```python
from build123d import *

# Parameters (mm, degrees)
PAD_DEPTH    = 15
SKETCH001_R  = 2
POCKET_DEPTH = 5
CHAMFER_SIZE = 1
FILLET_R     = 1


with BuildPart() as part:
    # Sketch → Pad (new body)
    with BuildSketch(Plane.XY):
        with BuildLine():
            Line((13, -10), (-35, -10))
            ThreePointArc((-35, 15), (-47.5, 2.5), (-35, -10))
            Line((-35, 15), (0, 15))
            Line((0, 15), (0, 0))
            Line((0, 0), (-5, 0))
            Line((-5, 0), (-5, 10))
            Line((-5, 10), (-35, 10))
            ThreePointArc((-35, 10), (-42.499997, 2.5), (-35, -5))
            Line((-35, -5), (13, -5))
            Line((13, -5), (13, -10))
        make_face()
    extrude(amount=PAD_DEPTH)

    # Sketch001 (on Face9 of Pad) → Pocket (cut)
    with BuildSketch(Plane(origin=(0, -5, 0), x_dir=(-1, 0, 0), z_dir=(0, 1, 0))):
        with Locations((-8, 7.5)):
            Circle(SKETCH001_R)
    extrude(amount=-POCKET_DEPTH, mode=Mode.SUBTRACT)

    # Chamfer
    chamfer_edges = [part.edges().sort_by_distance(p)[0] for p in [
        (10, -5, 7.5),
    ]]
    chamfer(chamfer_edges, length=CHAMFER_SIZE)

    # Fillet
    fillet_edges = [part.edges().sort_by_distance(p)[0] for p in [
        (-11, -10, 0),
        (13, -7.5, 0),
        (-11, -5, 0),
        (-20, 10, 0),
        (-5, 5, 0),
        (-2.5, 0, 0),
        (0, 7.5, 0),
        (13, -5, 7.5),
        (-11, -5, 15),
        (-17.5, 15, 0),
        (0, 15, 7.5),
        (-17.5, 15, 15),
        (-47.5, 2.5, 0),
        (-42.499997, 2.5, 0),
        (-47.5, 2.5, 15),
        (-20, 10, 15),
        (-42.499997, 2.5, 15),
        (-5, 5, 15),
        (-2.5, 0, 15),
        (0, 7.5, 15),
        (13, -7.5, 15),
        (-11, -10, 15),
        (-5, 0, 7.5),
        (0, 0, 7.5),
        (13, -10, 7.5),
    ]]
    fillet(fillet_edges, radius=FILLET_R)


solid = part.part
```
Part model, mm, in its own coordinate system. A direction names the side the tool comes from. Coordinates: 2 decimals unless noted, no trailing zeros. Loops run counter-clockwise (first coordinate to the right, second up) from the corner with the lowest first, then second, coordinate; pieces in that order, holes last. Notation, with made-up numbers: (-31.75, -9.5) - (16.25, -9.5) arc R12 cw to (16.25, 11.5) - close; hole circle Ø6 at (34.25, 34). An arc over 180 degrees is marked (long way). Write item = value, one per line. Start each with the question number.
Item 1: Cut at B-B, the plane y = 2.5. Give the cut face in (x, z).
Item 2: Cut at C-C, the plane x = -14.5. Give the cut face in (y, z), and give its area (3 significant figures).
Item 3: Cut at D-D, the plane z = 11.25. Give the cut face in (x, y), and give its area (3 significant figures).
Item 4: Wall check: L1, parallel to Y at x = -19, z = 8.25; L2, parallel to Z at x = 8, y = -7.8; L3, parallel to X at y = 2.75, z = 2.25. Give the ranges that are in metal, low to high. Write a range as from..to.
Item 5: Flat gauge pins, fed straight in: pin 1 Ø4.5 at (y, z) = (6.5, 7) entering from -X; pin 2 Ø6.5 at (y, z) = (9.5, 6) entering from +X. Where does each tip first touch, or does it go through?
Item 6: Mould opens along X. For faces 4 (the flat face through (-18, 15, 7)), 5 (the flat face through (0, 8, 7)), 6 (the cylindrical face through (9.474, -7.972, 8.852)), 7 (the cylindrical face through (-47.497, 2.775, 7.409)) say: released by +X, released by -X, zero draft, split by the parting line, or undercut.
Item 7: Cut at A-A, the plane z = 7.5. Give the cut face in (x, y), and give its area (3 significant figures).
Item 8: 3-axis set-ups, long thin cutter, end or side, ignore diameter. For faces 1 (the cylindrical face through (-42.5, 2.66, 7.41)), 2 (the flat face through (-12, -5, 7)), 3 (the flat face through (-11, -10, 7)): which of +Z, -Z, +X, -X, +Y, -Y reach the whole face in a straight line?
The answers:
q1.outline = (-47.5, 1) arc R1 ccw to (-46.5, 0) - (-43.5, 0) arc R1 ccw to (-42.5, 1) - (-42.5, 14) arc R1 ccw to (-43.5, 15) - (-46.5, 15) arc R1 ccw to (-47.5, 14) - close; (-5, 1) arc R1 ccw to (-4, 0) - (-1, 0) arc R1 ccw to (0, 1) - (0, 14) arc R1 ccw to (-1, 15) - (-4, 15) arc R1 ccw to (-5, 14) - close
q2.outline = (-10, 1) arc R1 ccw to (-9, 0) - (-6, 0) arc R1 ccw to (-5, 1) - (-5, 14) arc R1 ccw to (-6, 15) - (-9, 15) arc R1 ccw to (-10, 14) - close; (10, 1) arc R1 ccw to (11, 0) - (14, 0) arc R1 ccw to (15, 1) - (15, 14) arc R1 ccw to (14, 15) - (11, 15) arc R1 ccw to (10, 14) - close
q2.area = 148 mm2
q3.outline = (-35, -10) - (12, -10) arc R1 ccw to (13, -9) - (13, -6) arc R1 ccw to (12, -5) - (-35, -5) arc R7.5 cw to (-35, 10) - (-5, 10) - (-5, 1) arc R1 ccw to (-4, 0) - (-1, 0) arc R1 ccw to (0, 1) - (0, 14) arc R1 ccw to (-1, 15) - (-35, 15) arc R12.5 ccw to start
q3.area = 621 mm2
q4.L1 = -10..-5, 10..15
q4.L2 = 0..5.5, 9.5..15
q4.L3 = -47.5..-42.5, -5..0
q5.pin_1 = -47.38
q5.pin_2 = 0
q6.face_4 = zero draft
q6.face_5 = released by +X
q6.face_6 = undercut
q6.face_7 = released by -X
q7.outline = (-35, -10) - (6, -10) - (6, -6) - (5, -5) - (-35, -5) arc R7.5 cw to (-35, 10) - (-5, 10) - (-5, 1) arc R1 ccw to (-4, 0) - (-1, 0) arc R1 ccw to (0, 1) - (0, 14) arc R1 ccw to (-1, 15) - (-35, 15) arc R12.5 ccw to start; (10, -10) - (12, -10) arc R1 ccw to (13, -9) - (13, -6) arc R1 ccw to (12, -5) - (11, -5) - (10, -6) - close
q7.area = 600 mm2
q8.face_1 = +Z, -Z
q8.face_2 = +Z, -Z, +X
q8.face_3 = +Z, -Z, +X, -X, -Y
